```python
from build123d import *

# Parameters (mm, degrees)
F1_DEPTH  = 25.4
F3_DEPTH  = 15.24
F5_DEPTH  = 254
F6_W      = 12.7
F6_H      = 13.51927
F7_DEPTH  = 50.8
F9_DEPTH  = 12.7
F11_DEPTH = 50.8
F12_R     = 5.715
F13_DEPTH = 15.24


with BuildPart() as f1:
    # F0 (on Top) → F1 (new body)
    with BuildSketch(Plane.XY):
        with BuildLine():
            Line((-86.490609, -5.174935), (-88.820125, -5.174935))
            ThreePointArc((-88.820125, -5.174935), (-100.623355, -7.544352), (-88.610892, -6.749934))
            Line((-88.610892, -6.749934), (323.504108, -6.749934))
            ThreePointArc((323.504108, -6.749934), (335.516571, -7.544352), (323.713342, -5.174935))
            Line((323.713342, -5.174935), (-86.490609, -5.174935))
        make_face()
    extrude(amount=F1_DEPTH)

    # F2 (on face) → F3 (cut)
    with BuildSketch(Plane(origin=(0, 0, 0), x_dir=(1, 0, 0), z_dir=(0, 0, -1))):
        Polygon((323.504108, 5.174935), (323.504108, 6.749934), (-88.610892, 6.749934), (-88.820125, 5.174935), align=None)
    extrude(amount=-F3_DEPTH, mode=Mode.SUBTRACT)

    # F4 (on face) → F5 (join)
    with BuildSketch(Plane.XZ.offset(6.749934)):
        Polygon((123.796608, 25.4), (117.446608, 25.4), (111.096608, 25.4), (111.096608, 15.24), (123.796608, 15.24), align=None)
    extrude(amount=F5_DEPTH)

    # F6 (on face) → F7 (join)
    with BuildSketch(Plane.XY.offset(25.4)):
        with Locations((117.446608, -253.990299)):
            Rectangle(F6_W, F6_H)
    extrude(amount=F7_DEPTH)

    # F8 (on face) → F9 (join)
    with BuildSketch(Plane.XY.offset(76.2)):
        Polygon((168.246608, -247.230664), (111.096608, -247.230664), (66.646608, -247.230664), (66.646608, -260.749934), (168.246608, -260.749934), align=None)
    extrude(amount=F9_DEPTH)

    # F10 (on face) → F11 (join)
    with BuildSketch(Plane.XZ.offset(260.749934)):
        Polygon((66.646608, 88.9), (66.646608, 76.2), (111.096608, 76.2), (123.796608, 76.2), (168.246608, 76.2), (168.246608, 88.9), align=None)
    extrude(amount=F11_DEPTH)

    # F12 (on face) → F13 (join)
    with BuildSketch(Plane(origin=(0, 0, 76.2), x_dir=(1, 0, 0), z_dir=(0, 0, -1))):
        with Locations((74.153578, 303.118765)):
            Circle(F12_R)
        with Locations((160.739638, 303.118765)):
            Circle(F12_R)
    extrude(amount=F13_DEPTH)


solid = f1.part
```
Can you work these out from the model? Positions are in its coordinate system, mm. A direction names the side the tool comes from. Coordinates: 2 decimals unless noted, no trailing zeros. Loops run counter-clockwise (first coordinate to the right, second up) from the corner with the lowest first, then second, coordinate; pieces in that order, holes last. Notation, with made-up numbers: M 47,-21 L 89,-21 A9 ccw 89,-16 Z; hole C 73,57 d4. An arc over 180 degrees is marked long. Put each result on its own line as item: value. Start each with the question number.
(1) Will these pins go through, and if not, where does the flat tip stop? pin 1 Ø14 at (x, z) = (119, 37) entering from -Y; pin 2 Ø1 at (y, z) = (-34.5, 25) entering from -X; pin 3 Ø3.5 at (x, y) = (159, -305) entering from -Z.
(2) Imagine slicing it at D-D on x = -16. List the corners of the cut face in (y, z) for me.
(3) Which directions (+Z, -Z, +X, -X, +Y, -Y) give clear straight access to the entire face, cutting with the end or side of a thin tool? Please do faces 1 (the face through (222, -6.75, 20)), 2 (the face through (79.433, -300.93, 68.687)), 3 (the face through (117, -260.75, 45)), 4 (the face through (120, -5.175, 18)).
(4) Imagine slicing it at A-A on x = 73. List the corners of the cut face in (y, z) for me.
(5) I need wall thicknesses on probe 1 along Y at (x, z) = (-77, 23); probe 2 along X at (y, z) = (-133.5, 18); probe 3 along Z at (x, y) = (94, -292). Which ranges of each line are inside material? Lowest first, please.
(6) Imagine slicing it at C-C on y = -275.5. List the corners of the cut face in (x, z) for me.
Worked answers:
1. pin 1: stops at y = -260.75
1. pin 2: stops at x = 111.1
1. pin 3: stops at z = 60.96
2. outline: M -6.75,15.24 L -5.17,15.24 L -5.17,25.4 L -6.75,25.4 Z
3. face 1: +Z, -Z, -Y
3. face 2: -Z
3. face 3: -Z, +X, -X, -Y
3. face 4: +Z, -Z, +Y
4. outline: M -311.55,76.2 L -308.72,76.2 L -308.72,60.96 L -297.52,60.96 L -297.52,76.2 L -247.23,76.2 L -247.23,88.9 L -311.55,88.9 Z; M -6.75,15.24 L -5.17,15.24 L -5.17,25.4 L -6.75,25.4 Z
5. probe 1: y = -6.75 to -5.17
5. probe 2: x = 111.1 to 123.8
5. probe 3: z = 76.2 to 88.9
6. outline: M 66.65,76.2 L 168.25,76.2 L 168.25,88.9 L 66.65,88.9 Z
